from build123d import *

# Parameters (mm, degrees)
BOSS_EXTRUDE1_DEPTH     = 10
SKETCH2_W               = 8
SKETCH2_H               = 4.2
CUT_EXTRUDE1_DEPTH      = 4
CIRPATTERN4_START       = 3
CIRPATTERN4_DEPTH       = 4
CIRPATTERN4_2_OUTLINE_W = 4
CIRPATTERN4_2_OUTLINE_H = 4
CIRPATTERN4_2_DEPTH     = 4


# Read off the part's stored shape, not the designer's step: CirPattern4
with BuildPart() as part:
    # Sketch1 → Boss-Extrude1 (new body)
    with BuildSketch(Plane(origin=(0, 0, 0), x_dir=(1, 0, 0), z_dir=(0, 1, 0))):
        with BuildLine():
            Line((-4, 122), (-4, 117.932183902))
            ThreePointArc((-4, 117.932183902), (-102.190997647, 59), (-104.132267183, -55.501990336))
            Line((-104.132267183, -55.501990336), (-107.655099262, -57.535898385))
            Line((-107.655099262, -57.535898385), (-105.655099262, -61))
            Line((-105.655099262, -61), (-99.592921435, -57.5))
            ThreePointArc((-99.592921435, -57.5), (-99.592921435, 57.5), (0, 115))
            Line((0, 115), (0, 122))
            Line((0, 122), (-4, 122))
        make_face()
    extrude(amount=BOSS_EXTRUDE1_DEPTH)

    # Sketch2 → Cut-Extrude1 (cut)
    with BuildSketch(Plane(origin=(-105.655099262, 0, 61), x_dir=(0.4999999999999976, 0, 0.86602540378444), z_dir=(-0.8660254037844402, 0, 0.4999999999999977))):
        with Locations((0, 5)):
            Rectangle(SKETCH2_W, SKETCH2_H)
    extrude(amount=-CUT_EXTRUDE1_DEPTH, mode=Mode.SUBTRACT)

    # CirPattern4 outline → CirPattern4 (cut)
    with BuildSketch(Plane(origin=(0, 0, 0), x_dir=(1, 0, 0), z_dir=(0, 1, 0)).offset(CIRPATTERN4_START)):
        with BuildLine():
            ThreePointArc((-51.017828253, 103.063966547), (-39.505073194, 108.001616617), (-27.523562684, 111.657751622))
            Line((-27.523562684, 111.657751622), (-28.45299166, 114.518239882))
            ThreePointArc((-28.45299166, 114.518239882), (-40.431539839, 110.857072784), (-51.954522475, 105.946814933))
            Line((-51.954522475, 105.946814933), (-51.017828253, 103.063966547))
        make_face()
        with BuildLine():
            ThreePointArc((-80.369355178, 82.254281033), (-70.945892242, 90.507902273), (-60.680606447, 97.68758366))
            Line((-60.680606447, 97.68758366), (-62.448485416, 100.12086031))
            ThreePointArc((-62.448485416, 100.12086031), (-72.709398865, 92.93730853), (-82.151053465, 84.706578343))
            Line((-82.151053465, 84.706578343), (-80.369355178, 82.254281033))
        make_face()
        with BuildLine():
            ThreePointArc((-101.853769652, 53.392973393), (-95.442033049, 64.154643849), (-87.897809664, 74.15507438))
            Line((-87.897809664, 74.15507438), (-90.331086315, 75.922953349))
            ThreePointArc((-90.331086315, 75.922953349), (-97.869955334, 65.920192984), (-104.306066962, 55.17467168))
            Line((-104.306066962, 55.17467168), (-101.853769652, 53.392973393))
        make_face()
        with BuildLine():
            ThreePointArc((-113.368027495, 19.305189506), (-110.595642677, 31.521481894), (-106.510962851, 43.363749751))
            Line((-106.510962851, 43.363749751), (-109.371451112, 44.293178727))
            ThreePointArc((-109.371451112, 44.293178727), (-113.450318674, 32.450349656), (-116.250875881, 20.241883728))
            Line((-116.250875881, 20.241883728), (-113.368027495, 19.305189506))
        make_face()
        with BuildLine():
            ThreePointArc((-113.785032926, -16.672320837), (-114.923380235, -4.197222333), (-114.698080889, 8.327679163))
            Line((-114.698080889, 8.327679163), (-117.705776238, 8.327679163))
            ThreePointArc((-117.705776238, 8.327679163), (-117.925374368, -4.195959991), (-116.816239102, -16.672320837))
            Line((-116.816239102, -16.672320837), (-113.785032926, -16.672320837))
        make_face()
        with BuildLine():
            ThreePointArc((-103.063966547, -51.017828253), (-108.001616617, -39.505073194), (-111.657751621, -27.523562684))
            Line((-111.657751621, -27.523562684), (-114.518239882, -28.45299166))
            ThreePointArc((-114.518239882, -28.45299166), (-110.857072784, -40.431539839), (-105.946814933, -51.954522475))
            Line((-105.946814933, -51.954522475), (-103.063966547, -51.017828253))
        make_face()
    extrude(amount=CIRPATTERN4_DEPTH, mode=Mode.SUBTRACT)

    # CirPattern4 2 outline → CirPattern4 2 (add)
    with BuildSketch(Plane(origin=(0, 0, 0), x_dir=(1, 0, 0), z_dir=(0, 1, 0)).offset(CIRPATTERN4_START)):
        with Locations((2, 120)):
            Rectangle(CIRPATTERN4_2_OUTLINE_W, CIRPATTERN4_2_OUTLINE_H)
    extrude(amount=CIRPATTERN4_2_DEPTH)


solid = part.part
Work out the finished part from the listing and answer in its coordinate system (mm). A direction names the side the tool comes from. Give positions to 0.01 mm unless a question says otherwise; leave off trailing zeros. Order: outer loops, then holes, each group sorted by start corner. A loop starts at its lowest first (then second) coordinate and runs counter-clockwise, first axis right, second up. Notation, with made-up numbers: (82, -24) -> (110, -24) arc R15 cw to (110, 1) -> close; hole circle Ø8 at (10, 27.25). An arc over 180 degrees is marked (long way). One line per item, written item: value.
Item 1: Straight lines are drawn through the part: probe 1 along Z at (x, y) = (-8.5, 3.5); probe 2 along Z at (x, y) = (-106, 5.25); probe 3 along Z at (x, y) = (-102.5, 9.5). For each, find the intervals that lie inside material, in ascending order.
Answer sheet:
probe 1: -117.69 to -114.69
probe 2: -51.85 to -44.6
probe 3: -58.46 to -52.14, 52.14 to 59.18
Item 2: A tool of negligible diameter and unlimited length cuts with its end or side. For faces 4 (the flat face through (-116, 7, 4)), 5 (the flat face through (2, 5, -118)), 6 (the flat face through (-105, 2.9, 58)), from which of +Z, -Z, +X, -X, +Y, -Y can it reach the whole face along a straight path? Write none if from no direction.
Answer sheet:
face 4: +X, -X
face 5: +Z, +X, +Y, -Y
face 6: +Z, -X
Item 3: Find section A-A, the plane z = -91. Give the vertices of the cut face in (x, y).
Answer sheet:
outline: (-75.12, 0) -> (-70.31, 0) -> (-70.31, 3) -> (-75.12, 3) -> close; (-75.12, 7) -> (-70.31, 7) -> (-70.31, 10) -> (-75.12, 10) -> close
Item 4: Find section B-B, the plane x = -48. Give the vertices of the cut face in (y, z), plus the area to 3 significant figures.
Answer sheet:
outline: (0, -107.8) -> (3, -107.8) -> (3, -104.5) -> (0, -104.5) -> close; (7, -107.8) -> (10, -107.8) -> (10, -104.5) -> (7, -104.5) -> close
area: 19.8 mm²
Item 5: Find section C-C, the plane z = -47. Give the vertices of the cut face in (x, y), plus the area to 3 significant figures.
Answer sheet:
outline: (-108.24, 0) -> (-104.96, 0) -> (-104.96, 10) -> (-108.24, 10) -> close
area: 32.8 mm²
Item 6: Determine the mould class of faces 1 (the flat face through (0, 4.9, -117.7)), 2 (the flat face through (-110, 3, 40)), 3 (the flat face through (-1, 5, -122)) for opening direction Z: released by +Z, released by -Z, zero draft, split by the parting line, or undercut.
Answer sheet:
face 1: zero draft
face 2: undercut
face 3: released by -Z
Item 7: Flat-ended cylindrical pins translate along their axes: P1, Ø5, axis at x = -99.5, y = 7, coming from the +Z side; P2, Ø6, axis at y = 7, z = -39, coming from the +X side; P3, Ø3.5, axis at y = 5.5, z = -120.5, coming from the -X side. Find the tip coordinate at first contact, or state that the pin passes through.
Answer sheet:
P1: z = 58.89
P2: x = -107.06
P3: x = -4
